CAD build for the part. Positions are in the model's coordinates, mm. Round coordinates to 2 decimals unless told otherwise and drop trailing zeros. Loops run counter-clockwise (first coordinate to the right, second up) from the corner with the lowest first, then second, coordinate; pieces in that order, holes last. Notation, with made-up numbers: (77.5, 73.5) -> (89.5, 73.5) arc R34 ccw to (89.5, 108.5) -> close; hole circle Ø7 at (37.25, 36). An arc over 180 degrees is marked (long way). Answer as CSV lines item,"result".
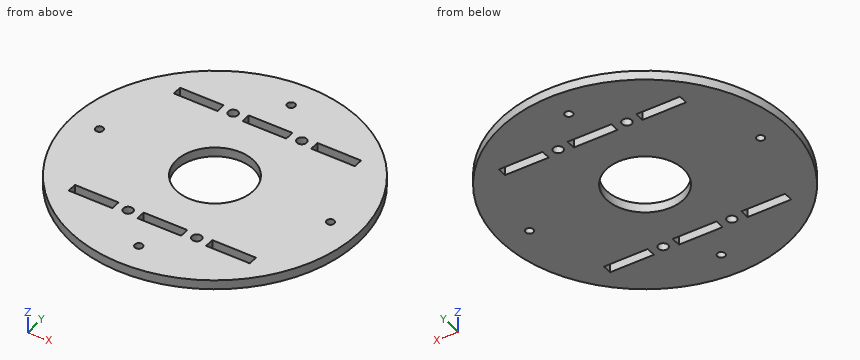
Autodesk Inventor part; units mm, degrees
ref_plane "YZ Plane" through (0, 0, 0) normal (1, 0, 0) x (0, 1, 0)
ref_plane "XZ Plane" through (0, 0, 0) normal (0, 1, 0) x (-1, 0, 0)
ref_plane "XY Plane" through (0, 0, 0) normal (0, 0, 1) x (1, 0, 0)
sketch "Sketch3" plane through (0, 0, 0) normal (0, 0, 1) x (1, 0, 0)
  circle A0 centre (0, 0) radius 46
  circle A1 centre (0, 0) radius 12.3
  circle A2 centre (0, 0) radius 37 construction
  circle A3 centre (0, 37) radius 1.25
  circle A4 centre (37, 0) radius 1.25
  circle A5 centre (0, -37) radius 1.25
  circle A6 centre (-37, 0) radius 1.25
  line L0 (-11, 25.5) -> (-11, -25.5) construction
  circle A7 centre (-11, 25.5) radius 1.55
  circle A8 centre (-11, -25.5) radius 1.55
  circle A9 centre (11, -25.5) radius 1.55
  line L1 (7, -27.05) -> (-7, -27.05)
  line L2 (-7, -27.05) -> (-7, -24.05)
  line L3 (-7, -24.05) -> (7, -24.05)
  line L4 (7, -24.05) -> (7, -27.05)
  line L5 (-15, -27.05) -> (-29, -27.05)
  line L6 (-29, -27.05) -> (-29, -24.05)
  line L7 (-29, -24.05) -> (-15, -24.05)
  line L8 (-15, -24.05) -> (-15, -27.05)
  line L9 (15, -27.05) -> (29, -27.05)
  line L10 (29, -27.05) -> (29, -24.05)
  line L11 (29, -24.05) -> (15, -24.05)
  line L12 (15, -24.05) -> (15, -27.05)
  line L13 (18.1239, 27.05) -> (15, 27.05)
  line L14 (7, 24) -> (-7, 24)
  line L15 (-7, 24) -> (-7, 27)
  line L16 (-7, 27) -> (7, 27)
  line L17 (7, 27) -> (7, 24)
  line L18 (-15, 24) -> (-29, 24)
  line L19 (-29, 24) -> (-29, 27)
  line L20 (-29, 27) -> (-15, 27)
  line L21 (-15, 27) -> (-15, 24)
  line L22 (15, 24) -> (29, 24)
  line L23 (29, 24) -> (29, 27)
  line L24 (29, 27) -> (15, 27)
  line L25 (15, 27) -> (15, 24)
  circle A10 centre (11, 25.5) radius 1.55
  line L26 (-46, -25.55) -> (46, -25.55) construction
  point P0 (46, 0)
  dimension "d74" = 92
  dimension "d32" = 2.5
  dimension "d33" = 2.5
  dimension "d34" = 2.5
  dimension "d35" = 2.5
  dimension "d45" = 3.1
  dimension "d46" = 3.1
  dimension "d47" = 3.1
  dimension "d50" = 14
  dimension "d51" = 4
  dimension "d53" = 14
  dimension "d54" = 4
  dimension "d57" = 14
  dimension "d58" = 14
  dimension "d59" = 14
  dimension "d60" = 3
  dimension "d61" = 14
  dimension "d64" = 3
  dimension "d65" = 3
  dimension "d71" = 1.5
  dimension "d72" = 1.5
  dimension "d75" = 74
  dimension "d78" = 24.6
  dimension "d80" = 3.1
  dimension "d81" = 25.5
  dimension "d82" = 25.5
  dimension "d83" = 22
  dimension "d84" = 11
  dimension "d87" = 4
  dimension "d91" = 22
  dimension "d92" = 1.5
  dimension "d93" = 1.5
  dimension "d94" = 1.5
  dimension "d95" = 1.5
  dimension "d96" = 1.5
  dimension "d97" = 1.5
  dimension "d98" = 4
extrude "Extrusion2" add sketch "Sketch3" along normal blind 3
properties part number "Base4"
Q1. Probe L1, parallel to Y at x = 0, z = 1.45; L2, parallel to Y at x = -11, z = 1.05; L3, parallel to Y at x = -4.5, z = 1.2. List the from-to ranges inside material, lowest first. Write a range as [from, to].
Results:
L1,"[-46, -38.25], [-35.75, -27.05], [-24.05, -12.3], [12.3, 24], [27, 35.75], [38.25, 46]"
L2,"[-44.67, -27.05], [-23.95, -5.5], [5.5, 23.95], [27.05, 44.67]"
L3,"[-45.78, -27.05], [-24.05, -11.45], [11.45, 24], [27, 45.78]"
Q2. Drop flat-ended pins along their axis: pin 1 Ø1.5 at (y, z) = (-25, 2) entering from +X; pin 2 Ø1.5 at (x, z) = (-21.5, 1) entering from -Y; pin 3 Ø1.5 at (y, z) = (6, 2) entering from -X. Give the stop position or say it passes through.
Results:
pin 1,"x = 39.09"
pin 2,"y = -41.05"
pin 3,"x = -45.7"
Q3. Slice it at A-A, the plane y = 0. Give the cut face in (x, z).
Results:
outline,"(-46, 0) -> (-38.25, 0) -> (-38.25, 3) -> (-46, 3) -> close; (-35.75, 0) -> (-12.3, 0) -> (-12.3, 3) -> (-35.75, 3) -> close; (12.3, 0) -> (35.75, 0) -> (35.75, 3) -> (12.3, 3) -> close; (38.25, 0) -> (46, 0) -> (46, 3) -> (38.25, 3) -> close"
Q4. Slice it at D-D, the plane x = 25.5. Give the cut face in (y, z), and give its area (3 significant figures).
Results:
outline,"(-38.29, 0) -> (-27.05, 0) -> (-27.05, 3) -> (-38.29, 3) -> close; (-24.05, 0) -> (24, 0) -> (24, 3) -> (-24.05, 3) -> close; (27, 0) -> (38.29, 0) -> (38.29, 3) -> (27, 3) -> close"
area,"212 mm2"
Q5. Slice it at C-C, the plane x = 37. Give the cut face in (y, z).
Results:
outline,"(-27.33, 0) -> (-1.25, 0) -> (-1.25, 3) -> (-27.33, 3) -> close; (1.25, 0) -> (27.33, 0) -> (27.33, 3) -> (1.25, 3) -> close"
Q6. Slice it at B-B, the plane z = 2.1. Count the separate pieces of the cut face and the enclosed holes in it, and give its area (3 significant figures).
Results:
separate pieces,"1"
enclosed holes,"15"
area,"5,870 mm2"
